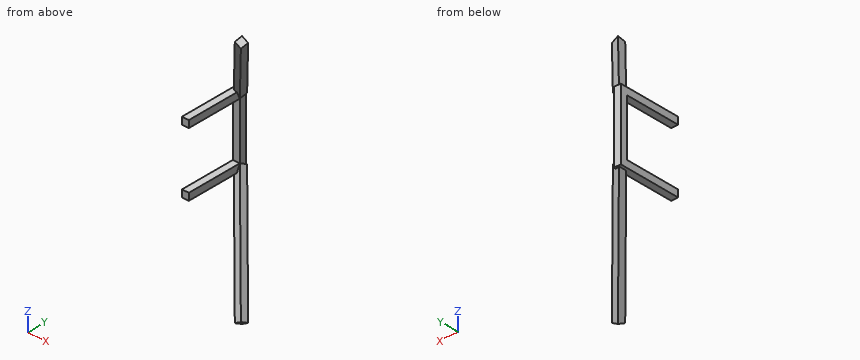
Autodesk Inventor part; units mm, degrees
ref_plane "YZ Plane" through (0, 0, 0) normal (1, 0, 0) x (0, 1, 0)
ref_plane "XZ Plane" through (0, 0, 0) normal (0, 1, 0) x (-1, 0, 0)
ref_plane "XY Plane" through (0, 0, 0) normal (0, 0, 1) x (1, 0, 0)
sketch "Sketch3" plane through (0, 0, 0) normal (0, 1, 0) x (-1, 0, 0)
  line L0 (311.15, 438.15) -> (-311.15, 438.15) construction
  line L1 (-311.15, 438.15) -> (-311.15, -438.15) construction
  line L2 (-311.15, -438.15) -> (311.15, -438.15) construction
  line L3 (311.15, -438.15) -> (311.15, 438.15) construction
  line L4 (0, -613.41) -> (0, 613.41) construction
  line L5 (435.61, 0) -> (-435.61, 0) construction
  line L6 (107.95, 438.15) -> (107.95, -438.15) construction
  line L7 (311.15, 102.1588) -> (-311.15, 102.1588) construction
  line L8 (311.15, -102.1588) -> (-311.15, -102.1588) construction
  line L9 (311.15, 127.5588) -> (285.75, 127.5588)
  line L10 (285.75, 127.5588) -> (285.75, 102.1588)
  line L11 (285.75, 102.1588) -> (311.15, 102.1588)
  line L12 (311.15, 102.1588) -> (311.15, 127.5588)
  line L13 (311.15, -102.1588) -> (285.75, -102.1588)
  line L14 (285.75, -102.1588) -> (285.75, -127.5588)
  line L15 (285.75, -127.5588) -> (311.15, -127.5588)
  line L16 (311.15, -127.5588) -> (311.15, -102.1588)
  point P0 (0, 0)
  dimension "d8" = 876.3
  dimension "d9" = 622.3
  dimension "d10" = 203.2
  dimension "d11" = 204.3176
  dimension "d12" = 25.4
  dimension "d13" = 25.4
  dimension "d14" = 25.4
  dimension "d15" = 25.4
extrude "Extrusion1" add sketch "Sketch3" along normal blind 203.2
ref_plane "Work Plane1" through (-285.75, 203.2, 127.5588) normal (0.8678585, 0, -0.4968114) x (0.4320296, -0.4937482, 0.7546941)
sketch "Sketch4" plane through (-285.75, 203.2, 127.5588) normal (0.8678585, 0, -0.4968114) x (0.4320296, -0.4937482, 0.7546941)
  line L0 (-19.8109, -14.5079) -> (410.9042, -25.3919)
  line L1 (410.9042, -25.3919) -> (411.5458, 0)
  line L2 (411.5458, 0) -> (-19.1692, 10.884)
  line L3 (-19.1692, 10.884) -> (-19.8109, -14.5079)
  line L4 (323.7574, 49.8449) -> (592.6095, -102.8051) construction
  line L5 (411.5458, 0) -> (-249.7926, 375.4977) construction
  point P0 (127.5142, 161.2687)
  dimension "d18" = 25.4
extrude "Extrusion2" add sketch "Sketch4" along normal mid plane 25.4
mirror "Mirror1" about plane through (0, 0, 0) normal (0, 0, 1) of "Extrusion2"
ref_plane "Work Plane2" through (-311.15, 203.2, -127.5588) normal (1, 0, 0) x (0, 0, 1)
sketch "Sketch5" plane through (-311.15, 203.2, -127.5588) normal (1, 0, 0) x (0, 0, 1)
  line L0 (0, 0) -> (255.1176, 0)
  line L1 (255.1176, 0) -> (255.1176, -25.4)
  line L2 (255.1176, -25.4) -> (0, -25.4)
  line L3 (0, -25.4) -> (0, 0)
  point P0 (127.5588, 203.2)
  dimension "d21" = 25.4
extrude "Extrusion3" add sketch "Sketch5" along normal blind 25.4
properties part number "Roll Bar"
CAD build for the part. Positions are in the model's coordinates, mm. Coordinates: 2 decimals unless noted, no trailing zeros. Order: outer loops, then holes, each group sorted by start corner. A loop starts at its lowest first (then second) coordinate and runs counter-clockwise, first axis right, second up.
(1) Saw through at C-C, the plane z = -20. Write the cut outline in (x, y), and give its area (3 significant figures).
Solution:
outline: (-311.15, 203.2) - (-285.75, 203.2) - (-285.75, 228.6) - (-311.15, 228.6) - close
area: 645 mm2
(2) Saw through at A-A, the plane x = -187. Write the cut outline in (y, z).
Solution:
outline: (73.24, -325.62) - (102.04, -325.62) - (125.77, -274.5) - (96.97, -274.5) - close; (73.24, 325.62) - (96.97, 274.5) - (125.77, 274.5) - (102.04, 325.62) - close
(3) Pin check, flat tips, straight feed: pin 1 Ø12.5 at (x, y) = (-298.5, 109) entering from -Z; pin 2 Ø7.5 at (x, y) = (-300.5, 121) entering from +Z; pin 3 Ø1 at (x, y) = (-278, 181) entering from -Z; pin 4 Ø6 at (y, z) = (169.5, 222.5) entering from +X. Stop position of each tip, or through.
Solution:
pin 1: stops at z = -127.56
pin 2: stops at z = 127.56
pin 3: stops at z = -167.53
pin 4: passes through
(4) Saw through at D-D, the plane z = 347. Write the cut outline in (x, y), and give its area (3 significant figures).
Solution:
outline: (-174.76, 60.06) - (-145.5, 52.29) - (-145.5, 81.09) - (-174.76, 88.87) - close
area: 843 mm2
(5) Saw through at B-B, the plane y = 107.5. Write the cut outline in (x, z), and give its area (3 significant figures).
Solution:
outline: (-311.15, -127.56) - (-285.75, -127.56) - (-285.75, -102.16) - (-311.15, -102.16) - close; (-311.15, 102.16) - (-285.75, 102.16) - (-285.75, 127.56) - (-311.15, 127.56) - close; (-218.83, -270.02) - (-192.07, -316.76) - (-170.03, -304.15) - (-196.78, -257.41) - close; (-218.83, 270.02) - (-196.78, 257.41) - (-170.03, 304.15) - (-192.07, 316.76) - close
area: 4,030 mm2
(6) Drill centre lines: L1, parallel to Z at x = -187.5, y = 100.5; L2, parallel to Z at x = -180.5, y = 83.5; L3, parallel to Y at x = -134, z = 394. Where is each one in solid material? Low to high.
Solution:
L1: z = -324.75 to -273.62, 273.62 to 324.75
L2: z = -336.98 to -299.79, 299.79 to 336.98
L3: y = 27.41 to 56.22
